Read the model definition and answer for the solid it produces. Units are mm, in the model's axes. Give positions to 0.01 mm unless a question says otherwise; leave off trailing zeros. Order: outer loops, then holes, each group sorted by start corner. A loop starts at its lowest first (then second) coordinate and runs counter-clockwise, first axis right, second up. Notation, with made-up numbers: (-27, -16.5) -> (-19, -16.5) arc R23 ccw to (-19, 3.5) -> close; hole circle Ø11 at (68, -18.5). An arc over 180 degrees is marked (long way). Use one line per item in the form item = value.
```python
from build123d import *

# Parameters (mm, degrees)
SKETCH1_W           = 111.5
SKETCH1_H           = 193
BOSS_EXTRUDE1_DEPTH = 6.1
SKETCH2_W           = 4
SKETCH2_H           = 6
SKETCH2_R           = 0.5
SKETCH2_W_2         = 6
SKETCH2_H_2         = 4
BOSS_EXTRUDE2_DEPTH = 2.4


with BuildPart() as part:
    # Sketch1 → Boss-Extrude1 (new body)
    with BuildSketch(Plane.XY):
        with Locations((55.75, 96.5)):
            Rectangle(SKETCH1_W, SKETCH1_H)
    extrude(amount=BOSS_EXTRUDE1_DEPTH)

    # Sketch2 → Boss-Extrude2 (add)
    with BuildSketch(Plane.XY.offset(6.1)):
        with Locations((22, 156.5)):
            Rectangle(SKETCH2_W, SKETCH2_H)
        with Locations((22, 156.5)):
            Circle(SKETCH2_R, mode=Mode.SUBTRACT)
        Polygon((87.5, 33), (85.5, 33), (85.5, 27), (89.5, 27), (89.5, 33), align=None)
        with Locations((87.5, 30)):
            Circle(SKETCH2_R, mode=Mode.SUBTRACT)
        with Locations((22, 30)):
            Rectangle(SKETCH2_W, SKETCH2_H)
        with Locations((22, 30)):
            Circle(SKETCH2_R, mode=Mode.SUBTRACT)
        with Locations((87.5, 156.5)):
            Rectangle(SKETCH2_W, SKETCH2_H)
        with Locations((87.5, 156.5)):
            Circle(SKETCH2_R, mode=Mode.SUBTRACT)
        with Locations((26, 58)):
            Rectangle(SKETCH2_W_2, SKETCH2_H_2)
        with Locations((26, 58)):
            Circle(SKETCH2_R, mode=Mode.SUBTRACT)
        with Locations((66.5, 116)):
            Rectangle(SKETCH2_W_2, SKETCH2_H_2)
        with Locations((66.5, 116)):
            Circle(SKETCH2_R, mode=Mode.SUBTRACT)
    extrude(amount=BOSS_EXTRUDE2_DEPTH)


solid = part.part
```
Item 1: The part is cut by section B-B on y = 106. Give the vertices of the cut face in (x, z).
Checks:
outline = (0, 0) -> (111.5, 0) -> (111.5, 6.1) -> (0, 6.1) -> close
Item 2: Straight lines are drawn through the part: L1, parallel to X at y = 156.5, z = 7.65; L2, parallel to Y at x = 22, z = 7.9; L3, parallel to Z at x = 82, y = 157.5. For each, find the intervals that lie inside material, in ascending order. Write a range as from..to.
Checks:
L1 = 20..21.5, 22.5..24, 85.5..87, 88..89.5
L2 = 27..29.5, 30.5..33, 153.5..156, 157..159.5
L3 = 0..6.1
Item 3: Given pin 1 Ø2.5 at (y, z) = (156.5, 8) entering from +X; pin 2 Ø1 at (x, y) = (45, 103.5) entering from +Z; pin 3 Ø1.9 at (y, z) = (31, 7.5) entering from -X, each flat-ended and moving along its own axis, determine where each tip first touches the part or whether it passes through.
Checks:
pin_1 = 89.5
pin_2 = 6.1
pin_3 = 20
Item 4: The part is cut by section A-A on x = 103. Give the vertices of the cut face in (y, z).
Checks:
outline = (0, 0) -> (193, 0) -> (193, 6.1) -> (0, 6.1) -> close
